Design review of the part built by this model. Coordinates are the model's own, in mm. A direction names the side the tool comes from. Give positions to 0.01 mm unless a question says otherwise; leave off trailing zeros. Loops run counter-clockwise (first coordinate to the right, second up) from the corner with the lowest first, then second, coordinate; pieces in that order, holes last. Notation, with made-up numbers: (28.5, -36) - (41.5, -36) arc R19 ccw to (41.5, -18) - close; hole circle Ø8 at (62, 34.5). An arc over 180 degrees is marked (long way). Put each result on its own line as item: value. Start each with the question number.
```python
from build123d import *

# Parameters (mm, degrees)
F0_W     = 5.842
F0_H     = 12.7
F0_R     = 3.175
F1_DEPTH = 25.4


with BuildPart() as f1:
    # F0 (on Front) → F1 (new body)
    with BuildSketch(Plane.XZ):
        Polygon((5.842, 12.7), (5.842, 0), (66.294, 0), (66.294, 12.7), (56.134, 12.7), (56.134, 10.16), (10.16, 10.16), (10.16, 12.7), align=None)
        with Locations((2.921, 6.35)):
            Rectangle(F0_W, F0_H)
        with BuildLine():
            Line((-0.9398, 0), (0, 0))
            Line((0, 0), (0, 12.7))
            Line((0, 12.7), (5.842, 12.7))
            Line((5.842, 12.7), (5.842, 15.24))
            Line((5.842, 15.24), (-0.508, 15.24))
            Line((-0.508, 15.24), (-10.88063, 3.847543))
            ThreePointArc((-10.88063, 3.847543), (-4.591961, 5.329721), (-0.9398, 0))
        make_face()
        with BuildLine():
            Line((5.842, 0), (0, 0))
            Line((0, 0), (-0.9398, 0))
            ThreePointArc((-0.9398, 0), (-3.195791, -4.549339), (-8.182663, -5.506983))
            Line((-8.182663, -5.506983), (5.842, -9.398))
            Line((5.842, -9.398), (5.842, 0))
        make_face()
        with BuildLine():
            ThreePointArc((-8.182663, -5.506983), (-3.195791, -4.549339), (-0.9398, 0))
            ThreePointArc((-0.9398, 0), (-4.591961, 5.329721), (-10.88063, 3.847543))
            ThreePointArc((-10.88063, 3.847543), (-12.145978, -1.583727), (-8.182663, -5.506983))
        make_face()
        with Locations((-6.6548, 0)):
            Circle(F0_R, mode=Mode.SUBTRACT)
    extrude(amount=F1_DEPTH)


solid = f1.part
```
Item 1: Mouldability with a two-part tool opening along X and no side actions: class faces 1 (the flat face through (5.842, -13, 14)), 2 (the flat face through (10.16, -13, 11)), 3 (the flat face through (26, -25.4, 6)) as pulls with the +X half, pulls with the -X half, needs draft (parallel to the pull), parting line crosses it, or undercut.
Item 2: For P1, Ø2, axis at y = -19, z = 11, coming from the -X side; P2, Ø5, axis at x = 59, y = -8, coming from the +Z side; P3, Ø12.5, axis at x = 35, y = -19, coming from the +Z side, all flat-tipped, find the tip position at first contact; note any pin that passes through.
Item 3: Consider section D-D (x = 36). State the section outline as (y, z) points, plus the area to 3 significant figures.
Item 4: Consider section B-B (x = -7). State the section outline as (y, z) points, plus the area to 3 significant figures.
Item 5: For L1, parallel to Z at x = 35.5, y = -19; L2, parallel to Z at x = 8, y = -4; L3, parallel to X at y = -1.25, z = -1.5, list the stretches that pass through material, from the lowest coordinate up. Write a range as from..to.
Item 6: Machinability: for faces 4 (the flat face through (3, -13, 15.24)), 5 (the flat face through (33, -13, 10.16)), 6 (the flat face through (61, -13, 12.7)), 7 (the flat face through (5.842, -13, -5)), which of the approach directions +Z, -Z, +X, -X, +Y, -Y give a long, thin tool a straight path to every point of the face, cutting with its end or side? Answer none if there is none.
Item 7: Consider section C-C (z = 2.25). State the section outline as (x, y) points, plus the area to 3 significant figures.
Item 8: Consider section A-A (y = -4). State the section outline as (x, z) points (3 decimals), plus the area to 3 significant figures.
Geometry says:
1. face 1: pulls with the +X half
1. face 2: undercut
1. face 3: needs draft
2. P1: stops at x = -5.28
2. P2: stops at z = 12.7
2. P3: stops at z = 10.16
3. outline: (-25.4, 0) - (0, 0) - (0, 10.16) - (-25.4, 10.16) - close
3. area: 258 mm2
4. outline: (-25.4, -5.84) - (0, -5.84) - (0, -3.16) - (-25.4, -3.16) - close; (-25.4, 3.16) - (0, 3.16) - (0, 8.11) - (-25.4, 8.11) - close
4. area: 194 mm2
5. L1: z = 0..10.16
5. L2: z = 0..12.7
5. L3: x = -12.17..-9.45, -3.86..5.84
6. face 4: +Z, +X, -X, +Y, -Y
6. face 5: +Z, +Y, -Y
6. face 6: +Z, +X, +Y, -Y
6. face 7: -Z, +X, +Y, -Y
7. outline: (-11.91, -25.4) - (-8.89, -25.4) - (-8.89, 0) - (-11.91, 0) - close; (-4.41, -25.4) - (66.29, -25.4) - (66.29, 0) - (-4.41, 0) - close
7. area: 1,870 mm2
8. outline: (-10.881, 3.848) arc R5.715 ccw to (-8.183, -5.507) - (5.842, -9.398) - (5.842, 0) - (66.294, 0) - (66.294, 12.7) - (56.134, 12.7) - (56.134, 10.16) - (10.16, 10.16) - (10.16, 12.7) - (5.842, 12.7) - (5.842, 15.24) - (-0.508, 15.24) - close; hole circle Ø6.35 at (-6.655, 0)
8. area: 941 mm2
